```python
from build123d import *

# Parameters (mm, degrees)
F0_R      = 12
F0_R_2    = 11
F0_R_3    = 5
F0_R_4    = 4.1
F0_R_5    = 3
F1_DEPTH  = 2
F2_DEPTH  = 3.5
F3_SIZE   = 0.99999
F4_DEPTH  = 4.5
F5_DEPTH  = 7.5
F6_SIZE   = 1
F7_SIZE   = 0.5
F8_R      = 3
F8_R_2    = 2.5
F9_DEPTH  = 3
F10_R     = 4.1
F10_R_2   = 3.6
F11_DEPTH = 3


# Not quite as in the source:
# - a fillet or chamfer is up to 0.001 mm smaller than in the source, because OpenCascade refuses the exact size


with BuildPart() as f1:
    # F0 (on Top) → F1 (new body)
    with BuildSketch(Plane.XY):
        Circle(F0_R)
        Circle(F0_R_2, mode=Mode.SUBTRACT)
        Circle(F0_R_2)
        Circle(F0_R_3, mode=Mode.SUBTRACT)
        Circle(F0_R_3)
        Circle(F0_R_4, mode=Mode.SUBTRACT)
        Circle(F0_R_4)
        Circle(F0_R_5, mode=Mode.SUBTRACT)
        Circle(F0_R_5)
    extrude(amount=F1_DEPTH)

    # F0 (on Top) → F2 (join)
    with BuildSketch(Plane.XY):
        Circle(F0_R_2)
        Circle(F0_R_3, mode=Mode.SUBTRACT)
        Circle(F0_R_3)
        Circle(F0_R_4, mode=Mode.SUBTRACT)
        Circle(F0_R_4)
        Circle(F0_R_5, mode=Mode.SUBTRACT)
        Circle(F0_R_5)
    extrude(amount=F2_DEPTH)

    # F3 (size 1 in the source; OpenCascade refuses exactly that, so slightly less here)
    f3_edges = [f1.edges().sort_by_distance(p)[0] for p in [
        (-11, 0, 2),
    ]]
    chamfer(f3_edges, length=F3_SIZE)

    # F0 (on Top) → F4 (join)
    with BuildSketch(Plane.XY):
        Circle(F0_R_3)
        Circle(F0_R_4, mode=Mode.SUBTRACT)
        Circle(F0_R_4)
        Circle(F0_R_5, mode=Mode.SUBTRACT)
        Circle(F0_R_5)
    extrude(amount=F4_DEPTH)

    # F0 (on Top) → F5 (join)
    with BuildSketch(Plane.XY):
        Circle(F0_R_4)
        Circle(F0_R_5, mode=Mode.SUBTRACT)
    extrude(amount=F5_DEPTH)

    # F6
    f6_edges = [f1.edges().sort_by_distance(p)[0] for p in [
        (-12, 0, 0),
    ]]
    chamfer(f6_edges, length=F6_SIZE)

    # F7
    f7_edges = [f1.edges().sort_by_distance(p)[0] for p in [
        (-11, 0, 3.5),
    ]]
    chamfer(f7_edges, length=F7_SIZE)

    # F8 (on face) → F9 (join, through all)
    with BuildSketch(Plane.XY.offset(4.5)):
        Circle(F8_R)
        Circle(F8_R_2, mode=Mode.SUBTRACT)
    extrude(amount=F9_DEPTH)

    # F10 (on face) → F11 (cut, through all)
    with BuildSketch(Plane.XY.offset(7.5)):
        Circle(F10_R)
        Circle(F10_R_2, mode=Mode.SUBTRACT)
    extrude(amount=-F11_DEPTH, mode=Mode.SUBTRACT)


solid = f1.part
```
Model file for the job. Use its own axes, mm. A direction names the side the tool comes from. Give positions to 0.01 mm unless a question says otherwise; leave off trailing zeros. Write each loop counter-clockwise with the first axis right and the second up, starting at its lowest first coordinate (ties: lowest second). Pieces come first, ordered by that corner, then holes. Notation, with made-up numbers: (52.5, 18.25) -> (102.5, 18.25) arc R19 cw to (102.5, 35.25) -> close; hole circle Ø7 at (45.5, -4.75). An arc over 180 degrees is marked (long way). Use CSV: the item, a comma, the result in double quotes. Start each with the question number.
1) Cut at C-C on z = 1.5. List the corners of the cut face in (x, y).
2) Two-plate mould, pull along X, no slides. Class faces 1 (the flat face through (5, -2, 3.5)), 2 (the cylindrical face through (-1.08, -4.88, 3.99)), 3 (the flat face through (0, 0, 4.5)): released by +X, released by -X, zero draft, split by the parting line, or undercut.
3) Pin check, flat tips, straight feed: P1, Ø1.5, axis at x = 0.5, y = -1, coming from the +Z side; P2, Ø1.5, axis at x = -7, z = 1, coming from the +Y side; P3, Ø5, axis at x = 5.5, y = -2, coming from the -Z side; P4, Ø1.5, axis at y = -5.5, z = 1, coming from the -X side. Stop position of each tip, or through.
4) Cut at D-D on z = 5. List the corners of the cut face in (x, y), plus the area to 3 significant figures.
5) Tool access for faces 4 (the cylindrical face through (-0.54, -2.44, 5.98)), 5 (the flat face through (-0.9, 2.5, 7.5)): list every direction of +Z, -Z, +X, -X, +Y, -Y with a clear straight run to the whole face (end or side of a thin tool).
6) Drill centre lines: L1, parallel to Y at x = 0, z = 6.95; L2, parallel to Z at x = 8, y = -2.5; L3, parallel to Z at x = -4, y = 2.75. Where is each one in solid material? Low to high.
Final values:
1,outline,"circle Ø24 at (0, 0)"
2,face 1,"zero draft"
2,face 2,"split by the parting line"
2,face 3,"undercut"
3,P1,"stops at z = 4.5"
3,P2,"stops at y = 10.24"
3,P3,"stops at z = 0"
3,P4,"stops at x = -11.02"
4,outline,"circle Ø7.2 at (0, 0); hole circle Ø5 at (0, 0)"
4,area,"21.1 mm2"
5,face 4,"+Z"
5,face 5,"+Z, +X, -X, +Y, -Y"
6,L1,"y = -3.6 to -2.5, 2.5 to 3.6"
6,L2,"z = 0 to 3.5"
6,L3,"z = 0 to 4.5"
